Autodesk Inventor part; units mm, degrees
ref_plane "dp1_XY" through (12.7, 7.9057, 0) normal (0, 0, 1) x (1, 0, 0)
ref_plane "dp1_YZ" through (12.7, 7.9057, 0) normal (1, 0, 0) x (0, 1, 0)
ref_plane "dp1_ZX" through (12.7, 7.9057, 0) normal (0, 1, 0) x (0, 0, 1)
sketch "Sketch_2" plane through (0, 0, 0) normal (0, 0, 1) x (1, 0, 0)
  line L0 (12.7, 0) -> (0, 0)
  line L1 (0, 0) -> (0, 7.098)
  line L2 (0, 7.098) -> (0.8395, 7.9375)
  line L3 (0.8395, 7.9375) -> (6.6726, 7.9375)
  line L4 (6.6726, 7.9375) -> (7.5126, 7.0988)
  arc A0 (7.5126, 7.0988) -> (8.1407, 6.839) centre (8.1407, 7.728) ccw
  line L5 (8.1407, 6.839) -> (9.4234, 6.839)
  arc A1 (9.4234, 6.839) -> (10.3124, 7.7279) centre (9.4234, 7.7279) ccw
  line L6 (10.3124, 7.7279) -> (10.3124, 7.9057)
  line L7 (10.3124, 7.9057) -> (12.7, 7.9057)
  line L8 (12.7, 7.9057) -> (12.7, 0)
  line L9 (12.7, 0) -> (0, 0)
revolve "Revolution1" add sketch "Sketch_2" angle 360 about axis through (12.7, 0, 0) along (1, 0, 0)
thread "Thread1"
sketch "Sketch_3" plane through (0, 0, 0) normal (0, 0, 1) x (1, 0, 0)
  line L0 (41.275, 0) -> (12.7, 0)
  line L1 (12.7, 0) -> (12.7, 13.3731)
  line L2 (12.7, 13.3731) -> (13.462, 14.1351)
  line L3 (13.462, 14.1351) -> (34.8615, 14.1351)
  line L4 (34.8615, 14.1351) -> (34.8615, 12.846)
  line L5 (34.8615, 12.846) -> (35.6235, 12.846)
  line L6 (35.6235, 12.846) -> (36.3855, 13.608)
  line L7 (36.3855, 13.608) -> (40.513, 13.608)
  line L8 (40.513, 13.608) -> (41.275, 12.846)
  line L9 (41.275, 12.846) -> (41.275, 0)
  line L10 (41.275, 0) -> (12.7, 0)
revolve "Revolution2" add sketch "Sketch_3" angle 360 about axis through (41.275, 0, 0) along (1, 0, 0)
sketch "Sketch3" plane through (0, 0, 0) normal (-1, 0, 0) x (0, 0, 1)
  point P0 (0, 0)
hole "Hole1" at (0, 0, 0) direction (1, 0, 0) diameter 8.0264 depth 41.275 countersink diameter 9.5504 countersink angle 90
sketch "Sketch_40" plane through (0, 0, 0) normal (0, 1, 0) x (-1, 0, 0)
  line L0 (-27.0002, 14.1351) -> (-27.0002, 0)
  line L1 (-27.0002, 0) -> (-30.1752, 0)
  line L2 (-30.1752, 0) -> (-30.1752, 3.243)
  line L3 (-30.1752, 3.243) -> (-31.5423, 4.6101)
  line L4 (-31.5423, 4.6101) -> (-31.8397, 14.1351)
  line L5 (-31.8397, 14.1351) -> (-27.0002, 14.1351)
  line L6 (-27.0002, 14.1351) -> (-27.0002, 0)
revolve "Revolution3" cut sketch "Sketch_40" angle 360 about axis through (27.0002, 0, 14.1351) along (0, 0, 1)
sketch "Sketch_47" plane through (0, 0, 0) normal (0, 0, 1) x (1, 0, 0)
  line L0 (35.6235, 0) -> (34.8615, 0)
  line L1 (34.8615, 12.5921) -> (35.6235, 12.5921)
  line L2 (35.6235, 12.5921) -> (35.6235, 12.846)
  line L3 (35.6235, 12.846) -> (35.2425, 12.846)
  line L4 (35.2425, 12.846) -> (34.984, 13.1046)
  arc A0 (34.984, 13.2842) -> (34.984, 13.1046) centre (35.0738, 13.1944) ccw
  line L5 (34.984, 13.2842) -> (35.7508, 14.0509)
  line L6 (35.7508, 14.0509) -> (35.7508, 14.1351)
  line L7 (35.7508, 14.1351) -> (35.5476, 14.1351)
  line L8 (35.5476, 14.1351) -> (34.8615, 13.449)
  line L9 (34.8615, 13.449) -> (34.8615, 12.5921)
revolve "Revolution4" add sketch "Sketch_47" angle 360 about axis through (35.6235, 0, 0) along (1, 0, 0)
ref_plane "dp1_XY" through (12.7, 7.9057, 0) normal (0, 0, 1) x (1, 0, 0)
ref_plane "dp1_YZ" through (12.7, 7.9057, 0) normal (1, 0, 0) x (0, 1, 0)
ref_plane "dp1_ZX" through (12.7, 7.9057, 0) normal (0, 1, 0) x (0, 0, 1)
ref_plane "dp2_XY" through (12.7, -7.9057, 0) normal (0, 0, 1) x (1, 0, 0)
ref_plane "dp2_YZ" through (12.7, -7.9057, 0) normal (1, 0, 0) x (0, 1, 0)
ref_plane "dp2_ZX" through (12.7, -7.9057, 0) normal (0, 1, 0) x (0, 0, 1)
ref_plane "port_XY" through (27.0002, 0, 0) normal (0, 0, 1) x (1, 0, 0)
ref_plane "port_YZ" through (27.0002, 0, 0) normal (1, 0, 0) x (0, 1, 0)
ref_plane "port_ZX" through (27.0002, 0, 0) normal (0, 1, 0) x (0, 0, 1)
ref_plane "rod_guide_XY" through (0, 0, 0) normal (1, 0, 0) x (0, 0, -1)
ref_plane "rod_guide_YZ" through (0, 0, 0) normal (0, 0, -1) x (0, 1, 0)
ref_plane "rod_guide_ZX" through (0, 0, 0) normal (0, 1, 0) x (1, 0, 0)
ref_plane "s1_XY" through (10.3124, 0, 0) normal (0, 0, 1) x (1, 0, 0)
ref_plane "s1_YZ" through (10.3124, 0, 0) normal (1, 0, 0) x (0, 1, 0)
ref_plane "s1_ZX" through (10.3124, 0, 0) normal (0, 1, 0) x (0, 0, 1)
ref_plane "s2_XY" through (12.7, 0, 0) normal (0, 0, 1) x (1, 0, 0)
ref_plane "s2_YZ" through (12.7, 0, 0) normal (1, 0, 0) x (0, 1, 0)
ref_plane "s2_ZX" through (12.7, 0, 0) normal (0, 1, 0) x (0, 0, 1)
ref_plane "t1_XY" through (12.7, 0, 0) normal (1, 0, 0) x (0, 0, -1)
ref_plane "t1_YZ" through (12.7, 0, 0) normal (0, 0, -1) x (0, 1, 0)
ref_plane "t1_ZX" through (12.7, 0, 0) normal (0, 1, 0) x (1, 0, 0)
ref_plane "t111_XY" through (12.7, 0, 0) normal (1, 0, 0) x (0, 0, -1)
ref_plane "t111_YZ" through (12.7, 0, 0) normal (0, 0, -1) x (0, 1, 0)
ref_plane "t111_ZX" through (12.7, 0, 0) normal (0, 1, 0) x (1, 0, 0)
ref_plane "to_foot_bracket_XY" through (12.7, 0, 0) normal (1, 0, 0) x (0, 0, -1)
ref_plane "to_foot_bracket_YZ" through (12.7, 0, 0) normal (0, 0, -1) x (0, 1, 0)
ref_plane "to_foot_bracket_ZX" through (12.7, 0, 0) normal (0, 1, 0) x (1, 0, 0)
ref_plane "to_nut_XY" through (10.3124, 0, 0) normal (1, 0, 0) x (0, 0, -1)
ref_plane "to_nut_YZ" through (10.3124, 0, 0) normal (0, 0, -1) x (0, 1, 0)
ref_plane "to_nut_ZX" through (10.3124, 0, 0) normal (0, 1, 0) x (1, 0, 0)
ref_plane "to_rod_XY" through (0, 0, 0) normal (1, 0, 0) x (0, 0, -1)
ref_plane "to_rod_YZ" through (0, 0, 0) normal (0, 0, -1) x (0, 1, 0)
ref_plane "to_rod_ZX" through (0, 0, 0) normal (0, 1, 0) x (1, 0, 0)
ref_plane "to_screw_XY" through (27.0002, 10.2743, -7.0485) normal (0, 1, 0) x (1, 0, 0)
ref_plane "to_screw_YZ" through (27.0002, 10.2743, -7.0485) normal (1, 0, 0) x (0, 0, -1)
ref_plane "to_screw_ZX" through (27.0002, 10.2743, -7.0485) normal (0, 0, -1) x (0, 1, 0)
ref_plane "to_trunnion_brackets_XY" through (18.2118, 0, 0) normal (0, 1, 0) x (1, 0, 0)
ref_plane "to_trunnion_brackets_YZ" through (18.2118, 0, 0) normal (1, 0, 0) x (0, 0, -1)
ref_plane "to_trunnion_brackets_ZX" through (18.2118, 0, 0) normal (0, 0, -1) x (0, 1, 0)
ref_plane "to_trunnion_brackets1_XY" through (18.2118, 15.875, 0) normal (0, 1, 0) x (1, 0, 0)
ref_plane "to_trunnion_brackets1_YZ" through (18.2118, 15.875, 0) normal (1, 0, 0) x (0, 0, -1)
ref_plane "to_trunnion_brackets1_ZX" through (18.2118, 15.875, 0) normal (0, 0, -1) x (0, 1, 0)
ref_plane "to_trunnion_brackets2_XY" through (18.2118, -15.875, 0) normal (0, 1, 0) x (1, 0, 0)
ref_plane "to_trunnion_brackets2_YZ" through (18.2118, -15.875, 0) normal (1, 0, 0) x (0, 0, -1)
ref_plane "to_trunnion_brackets2_ZX" through (18.2118, -15.875, 0) normal (0, 0, -1) x (0, 1, 0)
ref_plane "to_tube_XY" through (35.6235, 0, 0) normal (1, 0, 0) x (0, 0, -1)
ref_plane "to_tube_YZ" through (35.6235, 0, 0) normal (0, 0, -1) x (0, 1, 0)
ref_plane "to_tube_ZX" through (35.6235, 0, 0) normal (0, 1, 0) x (1, 0, 0)
properties part number "09R000-0_rod_guide"
Model file for the job. Use its own axes, mm. A direction names the side the tool comes from. Coordinates: 2 decimals unless noted, no trailing zeros. Order: outer loops, then holes, each group sorted by start corner. A loop starts at its lowest first (then second) coordinate and runs counter-clockwise, first axis right, second up. Notation, with made-up numbers: (51, 81.5) -> (101, 81.5) arc R12 cw to (101, 102.5) -> close; hole circle Ø3 at (5.25, -26). An arc over 180 degrees is marked (long way). Answer as a JSON object with one key per item and string values. Group by question number.
1) Drill centre lines: L1, parallel to Z at x = 32, y = 0; L2, parallel to X at y = 10, z = -0.5 (3 decimals); L3, parallel to Z at x = 30, y = 0. Where is each one in solid material? Low to high.
2) Cut at C-C, the plane x = 38.5. Write the cut outline in (y, z), then the cut area to 3 significant figures.
3) Cut at B-B, the plane y = 1. Count the separate pieces of the cut face and the enclosed holes in it, then the cut area to 3 significant figures.
4) Flat gauge pins, fed straight in: pin 1 (6 mm diameter, centred on x = 36.5, z = 7, fed in from +Y); pin 2 (4 mm diameter, centred on x = 27, y = -8.5, fed in from +Z); pin 3 (1 mm diameter, centred on x = 4, y = -9, fed in from -Z); pin 4 (2 mm diameter, centred on x = 11, z = 0, fed in from -Y). Where does each tip first touch, or does it go through?
5) Pull direction X, two halves, no side cores. Call faces 5 (the face through (8.791, 6.523, 2.054)), 6 (the face through (21.3, -0.18, -4.01)), 7 (the face through (41.275, 3, 3)), 8 (the face through (26.26, -3.33, 3.48)): +X half, -X half, draft (parallel to the pull), parting line (faces both ways), or undercut.
6) Which spindle directions (+Z, -Z, +X, -X, +Y, -Y) get a long thin tool onto all of the face, cutting with end or side? Do faces 1 (the face through (35.44, -2.78, -12.54)), 2 (the face through (3.8, -1.72, -7.75)), 3 (the face through (0, 5, -1)), 4 (the face through (38.478, -2.95, -13.284)). Say none if no direction does.
7) Cut at A-A, the plane x = 18.5. Write the cut outline in (y, z), then the cut area to 3 significant figures.
Check values:
{
 "1": {"L1": "z = -14.14 to -4.01, 4.01 to 14.14", "L2": "x = 12.7 to 41.275", "L3": "z = -14.14 to -4.01"},
 "2": {"outline": "circle Ø27.22 at (0, 0); hole circle Ø8.03 at (0, 0)", "area": "531 mm²"},
 "3": {"separate pieces": "3", "enclosed holes": "0", "area": "575 mm²"},
 "4": {"pin 1": "stops at y = 13.53", "pin 2": "stops at z = 12.55", "pin 3": "passes through", "pin 4": "stops at y = -7.91"},
 "5": {"face 5": "undercut", "face 6": "draft", "face 7": "+X half", "face 8": "undercut"},
 "6": {"face 1": "none", "face 2": "-X", "face 3": "+Z, -Z, -X, +Y, -Y", "face 4": "+X"},
 "7": {"outline": "circle Ø28.27 at (0, 0); hole circle Ø8.03 at (0, 0)", "area": "577 mm²"}
}
